Source: CAD feature listing. Evaluate the final solid. Frame: model axes, mm. Face numbers are marked on the shaded views. A direction names the side the tool comes from. Give positions to 0.01 mm unless a question says otherwise; leave off trailing zeros. Order: outer loops, then holes, each group sorted by start corner. A loop starts at its lowest first (then second) coordinate and runs counter-clockwise, first axis right, second up. Notation, with made-up numbers: M 14.25,28 L 27.25,28 A18 ccw 27.25,51 Z; hole C 64.5,-31.75 d7. An arc over 180 degrees is marked long. Answer in a Markdown table with one row per item. Add a question column.
(1) Pin query (flat end, axial travel): P1, Ø7, axis at x = 0, z = 0, coming from the -Y side; P2, Ø2.5, axis at y = -5, z = 8.5, coming from the -X side; P3, Ø2, axis at x = -5, y = -7, coming from the -Z side; P4, Ø4, axis at x = -13.5, y = -2.5, coming from the -Z side. Return the tip coordinate at first contact, or that it passes through.
(2) Section query B-B, the plane y = -2. Return loops of the section in (x, z).
(3) Set-up query: the marked faces 1 and 2. Return all of +Z, -Z, +X, -X, +Y, -Y with unobstructed straight access to the full face (end or side cutting, diameter ignored); none if empty.
(4) Section query C-C, the plane x = -2.5. Return loops of the section in (y, z).
(5) Section query A-A, the plane z = 34.5. Return loops of the section in (x, y).
(6) Mould query, pull axis X, two halves, no side actions, for the marked faces 3, 4, 5 and 6. Classes: pulls with the +X half, pulls with the -X half, needs draft (parallel to the pull), parting line crosses it, or undercut.
(7) Section query D-D, the plane z = 21. Return loops of the section in (x, y), plus the area to 3 significant figures.
(8) Material intervals for line 1 along X through (y, z) = (-5.75, 0); line 2 along X through (y, z) = (-6.75, -4); line 3 along Z through (x, y) = (3, -0.25), sorted ascending.
from build123d import *

# Parameters (mm, degrees)
EXTRUDE_1_DEPTH     = 25
EXTRUDE_2_DEPTH     = 9
SKETCH_3_R          = 4.5
CUT_EXTRUDE_1_DEPTH = 9
SKETCH_5_W          = 14
SKETCH_5_H          = 9
EXTRUDE_3_DEPTH     = 15
EXTRUDE_4_DEPTH     = 9
SKETCH_7_R          = 4.5
CUT_EXTRUDE_2_DEPTH = 9
SKETCH_8_W          = 14
SKETCH_8_H          = 14
EXTRUDE_5_DEPTH     = 9
FILLET_1_R          = 10


with BuildPart() as part:
    # Sketch 1 → Extrude 1 (new body)
    with BuildSketch(Plane.XY):
        Polygon((0, 0), (7, 0), (7, -9), (-7, -9), (-7, 0), align=None)
    extrude(amount=EXTRUDE_1_DEPTH)

    # Sketch 2 → Extrude 2 (add)
    with BuildSketch(Plane(origin=(0, 0, 0), x_dir=(1, 0, 0), z_dir=(0, 1, 0))):
        with BuildLine():
            Line((7, 0), (-7, 0))
            ThreePointArc((-7, 0), (0, 7), (7, 0))
        make_face()
    extrude(amount=-EXTRUDE_2_DEPTH)

    # Sketch 3 → Cut-Extrude 1 (cut)
    with BuildSketch(Plane(origin=(0, 0, 0), x_dir=(1, 0, 0), z_dir=(0, 1, 0))):
        with Locations(Location((0, 0, 0), (0, 0, 270))):
            Circle(SKETCH_3_R)
    extrude(amount=-CUT_EXTRUDE_1_DEPTH, mode=Mode.SUBTRACT)



with BuildPart() as body_2:
    # Sketch 5 → Extrude 3 (new body)
    with BuildSketch(Plane.ZY.offset(7)):
        with Locations((32, -4.5)):
            Rectangle(SKETCH_5_W, SKETCH_5_H)
    extrude(amount=EXTRUDE_3_DEPTH)

    # Sketch 6 → Extrude 4 (add)
    with BuildSketch(Plane(origin=(0, 0, 0), x_dir=(1, 0, 0), z_dir=(0, 1, 0))):
        with BuildLine():
            Line((-22, -25), (-22, -39))
            ThreePointArc((-22, -39), (-29, -32), (-22, -25))
        make_face()
    extrude(amount=-EXTRUDE_4_DEPTH)

    # Sketch 7 → Cut-Extrude 2 (cut)
    with BuildSketch(Plane(origin=(0, 0, 0), x_dir=(1, 0, 0), z_dir=(0, 1, 0))):
        with Locations(Location((-22, -32, 0), (0, 0, 270))):
            Circle(SKETCH_7_R)
    extrude(amount=-CUT_EXTRUDE_2_DEPTH, mode=Mode.SUBTRACT)


with BuildPart() as part_1:
    add(part.part)

    add(body_2.part)  # Extrude 5 merges body 2
    # Sketch 8 → Extrude 5 (add)
    with BuildSketch(Plane(origin=(0, 0, 0), x_dir=(1, 0, 0), z_dir=(0, 1, 0))):
        with Locations((0, -32)):
            Rectangle(SKETCH_8_W, SKETCH_8_H)
    extrude(amount=-EXTRUDE_5_DEPTH)

    # Fillet 1
    fillet_1_edges = [part_1.edges().sort_by_distance(p)[0] for p in [
        (7, -4.5, 39),
        (-7, -4.5, 25),
    ]]
    fillet(fillet_1_edges, radius=FILLET_1_R)


solid = part_1.part
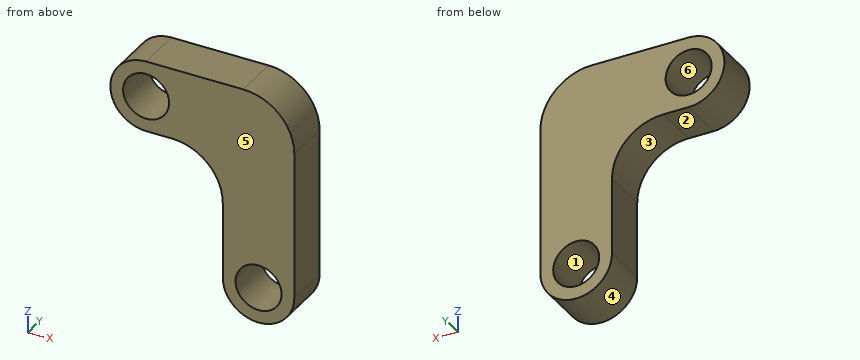
Values follow:
| question | item | result |
|---|---|---|
| 1 | P1 | passes through |
| 1 | P2 | stops at x = -7 |
| 1 | P3 | stops at z = -5.74 |
| 1 | P4 | stops at z = 23.35 |
| 2 | outline | M -22,25 L -17,25 A10 cw -7,15 L -7,0 A7 ccw 7,0 L 7,29 A10 ccw -3,39 L -22,39 A7 ccw Z; hole C -22,32 d9; hole C 0,0 d9 |
| 3 | face 1 | +Y, -Y |
| 3 | face 2 | -Z, -X, +Y, -Y |
| 4 | outline | M -9,-6.54 L 0,-6.54 L 0,-3.74 L -9,-3.74 Z; M -9,3.74 L 0,3.74 L 0,38.99 L -9,38.99 Z |
| 5 | outline | M -28.54,-9 L -25.74,-9 L -25.74,0 L -28.54,0 Z; M -18.26,-9 L 5.35,-9 L 5.35,0 L -18.26,0 Z |
| 6 | face 3 | pulls with the -X half |
| 6 | face 4 | parting line crosses it |
| 6 | face 5 | needs draft |
| 6 | face 6 | undercut |
| 7 | outline | M -9,-9 L 7,-9 L 7,0 L -9,0 Z |
| 7 | area | 144 mm² |
| 8 | line 1 | x = -7 to -4.5, 4.5 to 7 |
| 8 | line 2 | x = -5.74 to -2.06, 2.06 to 5.74 |
| 8 | line 3 | z = -6.32 to -3.35, 3.35 to 37 |
